For this review, take the finished solid that the model builds, in its own axes (mm). A direction names the side the tool comes from. Give positions to 0.01 mm unless a question says otherwise; leave off trailing zeros. Loops run counter-clockwise (first coordinate to the right, second up) from the corner with the lowest first, then second, coordinate; pieces in that order, holes last. Notation, with made-up numbers: (-12, 56) - (28, 56) arc R21 ccw to (28, 75) - close; hole circle Ø2 at (-15.75, 48). An arc over 180 degrees is marked (long way). Put each result on its own line as item: value.
Autodesk Inventor part; units mm, degrees
ref_plane "YZ Plane" through (0, 0, 0) normal (1, 0, 0) x (0, 1, 0)
ref_plane "XZ Plane" through (0, 0, 0) normal (0, 1, 0) x (-1, 0, 0)
ref_plane "XY Plane" through (0, 0, 0) normal (0, 0, 1) x (1, 0, 0)
sketch "Sketch1" plane through (0, 0, 0) normal (0, 0, 1) x (1, 0, 0)
  circle A0 centre (0, 0) radius 31.5
  line L0 (0, 0) -> (17.6777, 17.6777)
  line L1 (0, 0) -> (25, 0) construction
  circle A1 centre (17.6777, 17.6777) radius 3.1
  circle A2 centre (-6.4705, 24.1481) radius 3.1
  circle A3 centre (-24.1481, 6.4705) radius 3.1
  circle A4 centre (-17.6777, -17.6777) radius 3.1
  circle A5 centre (6.4705, -24.1481) radius 3.1
  circle A6 centre (24.1481, -6.4705) radius 3.1
  dimension "d0" = 63
  dimension "d1" = 25
  dimension "d2" = 45
  dimension "d3" = 6.2
  dimension "d6" = 360
extrude "Extrusion1" add sketch "Sketch1" along normal blind 10
sketch "Sketch2" plane through (0, 0, 10) normal (0, 0, 1) x (1, 0, 0)
  line L0 (12.5, -12.5) -> (-12.5, -12.5)
  line L1 (-12.5, -12.5) -> (-12.5, 12.5)
  line L2 (-12.5, 12.5) -> (12.5, 12.5)
  line L3 (12.5, 12.5) -> (12.5, -12.5)
  line L4 (12.5, -12.5) -> (-12.5, 12.5) construction
  line L5 (-12.5, -12.5) -> (12.5, 12.5) construction
  point P0 (0, 0)
  dimension "d10" = 25
  dimension "d11" = 25
extrude "Extrusion2" add sketch "Sketch2" along normal blind 50
sketch "Sketch4" plane through (0, 0, 60) normal (0, 0, 1) x (1, 0, 0)
  line L0 (7.5, -7.5) -> (-7.5, -7.5)
  line L1 (-7.5, -7.5) -> (-7.5, 7.5)
  line L2 (-7.5, 7.5) -> (7.5, 7.5)
  line L3 (7.5, 7.5) -> (7.5, -7.5)
  line L4 (7.5, -7.5) -> (-7.5, 7.5) construction
  line L5 (-7.5, -7.5) -> (7.5, 7.5) construction
  line L6 (6.5, 6.5) -> (-6.5, 6.5)
  line L7 (-6.5, 6.5) -> (-6.5, -6.5)
  line L8 (-6.5, -6.5) -> (6.5, -6.5)
  line L9 (6.5, -6.5) -> (6.5, 6.5)
  line L10 (-9.4383, 2.5) -> (11.9316, 2.5)
  line L11 (-9.4383, -2.5) -> (9.2053, -2.5)
  line L12 (-2.5, 9.4032) -> (-2.5, -10.6036)
  line L13 (2.5, 9.4032) -> (2.5, -9.3606)
  point P0 (0, 0)
  point P1 (2.5, 7.5)
  point P2 (2.5, 6.5)
  point P3 (6.5, 2.5)
  point P4 (7.5, 2.5)
  point P5 (2.5, -6.5)
  point P6 (2.5, -7.5)
  point P7 (7.5, -2.5)
  point P8 (6.5, -2.5)
  point P9 (-2.5, -7.5)
  point P10 (-2.5, -6.5)
  point P11 (-6.5, -2.5)
  point P12 (-7.5, -2.5)
  point P13 (-2.5, 6.5)
  point P14 (-2.5, 7.5)
  point P15 (-7.5, 2.5)
  point P16 (-6.5, 2.5)
  dimension "d27" = 15
  dimension "d28" = 15
  dimension "d29" = 1
  dimension "d30" = 18.7639
  dimension "d31" = 5
  dimension "d32" = 5
  dimension "d33" = 5
  dimension "d34" = 5
extrude "Extrusion4" add sketch "Sketch4" along normal blind 1 contours L0 L13 L8 L9 L11 L3 | L0 L1 L11 L7 L8 L12 | L10 L9 L6 L13 L2 L3 | L1 L2 L12 L6 L7 L10
properties part number "soporte p1"
1) Take a section at A-A on x = 23. State the section outline as (y, z) points.
Geometry check:
outline: (-21.52, 0) - (-9.35, 0) - (-9.35, 10) - (-21.52, 10) - close; (-3.59, 0) - (21.52, 0) - (21.52, 10) - (-3.59, 10) - close
2) Draft analysis for pull direction X (two halves, no side actions). For faces 1 (the face through (7, -6, 61)), 2 (the face through (27.105, -7.402, 4.93)), 3 (the face through (0, 0, 60)), 4 (the face through (-12.5, 0, 35)), state which applies: pulls with the +X half, pulls with the -X half, needs draft (parallel to the pull), parting line crosses it, or undercut.
Geometry check:
face 1: needs draft
face 2: undercut
face 3: undercut
face 4: pulls with the -X half
3) Take a section at C-C on y = -15.5. State the section outline as (x, z) points.
Geometry check:
outline: (-27.42, 0) - (-19.88, 0) - (-19.88, 10) - (-27.42, 10) - close; (-15.47, 0) - (27.42, 0) - (27.42, 10) - (-15.47, 10) - close
4) Insertion check: pin 1 Ø20 at (y, z) = (3.5, 31) entering from +X; pin 2 Ø0.5 at (y, z) = (-5.5, 60.5) entering from +X; pin 3 Ø1.1 at (y, z) = (5.5, 60.5) entering from -X; pin 4 Ø8 at (x, z) = (-18.5, 19) entering from +Y. Each pin has a flat end and moves straight along its axis. Give the tip position at first contact, or say it passes through.
Geometry check:
pin 1: stops at x = 12.5
pin 2: stops at x = 7.5
pin 3: stops at x = -12.5
pin 4: passes through
5) For faces 5 (the face through (-7, -6, 61)), 6 (the face through (0, -12.5, 35)), 7 (the face through (12.5, 0, 35)), 8 (the face through (0, 12.5, 35)), list the 3-axis set-ups (+Z, -Z, +X, -X, +Y, -Y) from which the entire face can be reached by the end or side of a thin tool; tool diameter is ignored.
Geometry check:
face 5: +Z, +X, -X, +Y, -Y
face 6: +Z, +X, -X, -Y
face 7: +Z, +X, +Y, -Y
face 8: +Z, +X, -X, +Y
6) Wall thickness on line 1 (Z direction, x = 10, y = 27); line 2 (X direction, y = -11.5, z = 45); line 3 (Y direction, x = -26, z = 4): over which ranges is each line inside the solid? List them lowest first.
Geometry check:
line 1: z = 0 to 10
line 2: x = -12.5 to 12.5
line 3: y = -17.78 to 3.98, 8.96 to 17.78
7) Take a section at B-B on z = 8.5. State the section outline as (x, y) points, and give its area (3 significant figures).
Geometry check:
outline: circle Ø63 at (0, 0); hole circle Ø6.2 at (-24.15, 6.47); hole circle Ø6.2 at (-17.68, -17.68); hole circle Ø6.2 at (-6.47, 24.15); hole circle Ø6.2 at (6.47, -24.15); hole circle Ø6.2 at (17.68, 17.68); hole circle Ø6.2 at (24.15, -6.47)
area: 2,940 mm²
8) Take a section at D-D on x = 0. State the section outline as (y, z) points, and give its area (3 significant figures).
Geometry check:
outline: (-31.5, 0) - (31.5, 0) - (31.5, 10) - (12.5, 10) - (12.5, 60) - (-12.5, 60) - (-12.5, 10) - (-31.5, 10) - close
area: 1,880 mm²
